For this review, take the finished solid that the model builds, in its own axes (mm). A direction names the side the tool comes from. Give positions to 0.01 mm unless a question says otherwise; leave off trailing zeros. Write each loop counter-clockwise with the first axis right and the second up, starting at its lowest first coordinate (ties: lowest second). Pieces come first, ordered by that corner, then holes.
1) For P1, Ø5, axis at x = 24.7, y = 6, coming from the -Z side; P2, Ø5.5, axis at x = 44.7, y = 4.7, coming from the -Z side; P3, Ø4, axis at x = 4.7, y = 143.3, coming from the -Z side, all flat-tipped, find the tip position at first contact; note any pin that passes through.
2) We need section A-A on x = 15. Give the boundary of the cut face in (y, z).
3) We need section B-B on y = 115.5. Give the boundary of the cut face in (x, z), and give its area (3 significant figures).
4) We need section C-C on y = 48. Give the boundary of the cut face in (x, z), and give its area (3 significant figures).
5) We need section D-D on z = 0.9. Give the number of separate pieces and of enclosed holes in the cut face, and give its area (3 significant figures).
6) Machinability: for faces 1 (the face through (25, 48, 2.1)), 2 (the face through (24, 148, 1)), which of the approach directions +Z, -Z, +X, -X, +Y, -Y give a long, thin tool a straight path to every point of the face, cutting with its end or side? Answer none if there is none.
7) Wall thickness on line 1 along X through (y, z) = (143.3, 2.85); line 2 along Y through (x, z) = (4.7, 2.9); line 3 along Y through (x, z) = (21, 0.3): over which ranges is each line inside the solid? List them lowest first.
8) Draft analysis for pull direction Y (two halves, no side actions). For faces 3 (the face through (4.32, 141.59, 2.8)), 4 (the face through (24, 0, 1)), 5 (the face through (42.95, 4.78, 2.8)), 6 (the face through (49.4, 73, 1)), state which applies: pulls with the +Y half, pulls with the -Y half, needs draft (parallel to the pull), parting line crosses it, or undercut.
from build123d import *

# Parameters (mm, degrees)
SKETCH_W     = 49.4
SKETCH_H     = 148
SKETCH_R     = 1.75
SKETCH_R_2   = 23.5
PAD_DEPTH    = 3
SKETCH001_R  = 3.1
POCKET_DEPTH = 2.1
CHAMFER_SIZE = 2.6


with BuildPart() as part:
    # Sketch → Pad (new body)
    with BuildSketch(Plane.XY):
        with Locations((24.7, 74)):
            Rectangle(SKETCH_W, SKETCH_H)
        with Locations((24.7, 126.745966)):
            Circle(SKETCH_R, mode=Mode.SUBTRACT)
        with Locations((24.7, 65.745966)):
            Circle(SKETCH_R, mode=Mode.SUBTRACT)
        with Locations((24.7, 96.245966)):
            Circle(SKETCH_R_2, mode=Mode.SUBTRACT)
        with Locations((4.7, 143.3)):
            Circle(SKETCH_R, mode=Mode.SUBTRACT)
        with Locations((44.7, 143.3)):
            Circle(SKETCH_R, mode=Mode.SUBTRACT)
        with Locations((4.7, 4.7)):
            Circle(SKETCH_R, mode=Mode.SUBTRACT)
        with Locations((44.7, 4.7)):
            Circle(SKETCH_R, mode=Mode.SUBTRACT)
    extrude(amount=PAD_DEPTH)

    # Sketch001 → Pocket (cut)
    with BuildSketch(Plane.XY):
        with Locations((24.7, 142)):
            Circle(SKETCH001_R)
        with Locations((24.7, 48)):
            Circle(SKETCH001_R)
        with Locations((24.7, 6)):
            Circle(SKETCH001_R)
    extrude(amount=POCKET_DEPTH, mode=Mode.SUBTRACT)

    # Chamfer
    chamfer_edges = [part.edges().sort_by_distance(p)[0] for p in [
        (42.95, 143.3, 0),
        (2.95, 143.3, 0),
        (2.95, 4.7, 0),
        (22.95, 65.745966, 0),
        (22.95, 126.745966, 0),
        (42.95, 4.7, 0),
    ]]
    chamfer(chamfer_edges, length=CHAMFER_SIZE)


solid = part.part
Results list:
1. P1: stops at z = 2.1
1. P2: stops at z = 1.6
1. P3: stops at z = 2.35
2. outline: (0, 0) - (74.84, 0) - (74.84, 3) - (0, 3) - close; (117.65, 0) - (148, 0) - (148, 3) - (117.65, 3) - close
3. outline: (0, 0) - (11.23, 0) - (11.23, 3) - (0, 3) - close; (38.17, 0) - (49.4, 0) - (49.4, 3) - (38.17, 3) - close
3. area: 67.4 mm2
4. outline: (0, 0) - (21.6, 0) - (21.6, 2.1) - (27.8, 2.1) - (27.8, 0) - (49.4, 0) - (49.4, 3) - (0, 3) - close
4. area: 135 mm2
5. separate pieces: 1
5. enclosed holes: 10
5. area: 5,260 mm2
6. face 1: -Z
6. face 2: +Z, -Z, +X, -X, +Y
7. line 1: x = 0 to 2.95, 6.45 to 42.95, 46.45 to 49.4
7. line 2: y = 0 to 2.95, 6.45 to 83.91, 108.58 to 141.55, 145.05 to 148
7. line 3: y = 0 to 64.1, 67.39 to 73.04, 119.45 to 125.1, 128.39 to 148
8. face 3: undercut
8. face 4: pulls with the -Y half
8. face 5: undercut
8. face 6: needs draft
